Read the model definition and answer for the solid it produces. Units are mm, in the model's axes. Round coordinates to 2 decimals unless told otherwise and drop trailing zeros. Write each loop counter-clockwise with the first axis right and the second up, starting at its lowest first coordinate (ties: lowest second). Pieces come first, ordered by that corner, then holes. Notation, with made-up numbers: (53.5, 70.25) - (82.5, 70.25) arc R20 cw to (82.5, 95.25) - close; hole circle Ø10 at (45.25, -6.75). An arc over 180 degrees is marked (long way). One line per item, written item: value. Start each with the question number.
(1) Find the intervals of material crossed by L1, parallel to Y at x = -194, z = 4.25; L2, parallel to Y at x = 176.5, z = 2.75; L3, parallel to Y at x = 102.5, z = 2.75, in increasing order.
(2) Flat-ended cylindrical pins translate along their axes: pin 1 Ø1.5 at (y, z) = (-174, 6.5) entering from -X; pin 2 Ø2 at (x, z) = (-128.5, 6.5) entering from -Y; pin 3 Ø3 at (x, z) = (-5.5, 3) entering from -Y. Find the tip coordinate at first contact, or state that the pin passes through.
(3) A cutting plane is placed at A-A, the plane y = 86. Determine the outline of the cut face in (x, z).
(4) A cutting plane is placed at B-B, the plane z = 4.25. State how many separate pieces and enclosed holes the cut face has, plus the area to 3 significant figures.
(5) The mould has two halves that part along X. Classify faces 1 (the face through (58.074, 138.231, 5.051)), 2 (the face through (-52.9, 129.55, 5.05)), 3 (the face through (-3, -52, 0)): +X half, -X half, draft (parallel to the pull), parting line (faces both ways), or undercut.
(6) A cutting plane is placed at C-C, the plane y = -62. Determine the outline of the cut face in (x, z), plus the area to 3 significant figures.
from build123d import *

# Parameters (mm, degrees)
SKETCH1_R           = 250
SKETCH1_R_2         = 40
BOSS_EXTRUDE1_DEPTH = 1.6
SKETCH3_R           = 250
SKETCH3_R_2         = 240
SKETCH3_R_3         = 50
SKETCH3_R_4         = 40
BOSS_EXTRUDE2_DEPTH = 7
RIB2_REACH          = 355.658
SKETCH4_WALLS_W     = 899.315940722
SKETCH4_WALLS_H     = 10
CIRPATTERN1_COUNT   = 8
EXTRUDE_THIN1_START = -7
SKETCH5_R           = 149.934912721
SKETCH5_R_2         = 139.934912721
EXTRUDE_THIN1_DEPTH = 7


with BuildPart() as part:
    # Sketch1 → Boss-Extrude1 (new body)
    with BuildSketch(Plane.XY):
        Circle(SKETCH1_R)
        Circle(SKETCH1_R_2, mode=Mode.SUBTRACT)
    extrude(amount=BOSS_EXTRUDE1_DEPTH)

    # Sketch3 → Boss-Extrude2 (add)
    # profile 1 of 2: a face of its own
    with BuildSketch(Plane.XY.offset(1.6)):
        Circle(SKETCH3_R)
        Circle(SKETCH3_R_2, mode=Mode.SUBTRACT)
    # profile 2 of 2: a face of its own
    with BuildSketch(Plane.XY.offset(1.6)):
        Circle(SKETCH3_R_3)
        Circle(SKETCH3_R_4, mode=Mode.SUBTRACT)
    extrude(amount=BOSS_EXTRUDE2_DEPTH)

    # Sketch4 walls → Rib2 (add, up to next)
    with BuildSketch(Plane.XY.offset(8.6), mode=Mode.PRIVATE) as rib2_sk1:
        with Locations((145, 0)):
            Rectangle(SKETCH4_WALLS_W, SKETCH4_WALLS_H)
    rib2_tool1 = extrude(rib2_sk1.sketch, amount=-RIB2_REACH, mode=Mode.PRIVATE) - part.part
    rib2 = rib2_tool1.solids().sort_by_distance((145, 0, 8.6))[0]
    add(rib2)

    # CirPattern1: Rib2 ×8 about axis
    cirpattern1_axis = Axis((0, 0, 0), (0, 0, 1))
    for i in range(1, CIRPATTERN1_COUNT):
        add(rib2.rotate(cirpattern1_axis, i * 360 / CIRPATTERN1_COUNT))

    # Sketch5 → Extrude-Thin1 (add)
    with BuildSketch(Plane.XY.offset(8.6).offset(EXTRUDE_THIN1_START)):
        Circle(SKETCH5_R)
        Circle(SKETCH5_R_2, mode=Mode.SUBTRACT)
    extrude(amount=EXTRUDE_THIN1_DEPTH)


solid = part.part
Here are the results:
1. L1: -157.68 to -141.29, -5 to 5, 141.29 to 157.68
1. L2: -177.05 to -162.63, -5 to 5, 162.63 to 177.05
1. L3: -228.02 to -217.01, -109.57 to -95.27, -5 to 5, 95.27 to 109.57, 217.01 to 228.02
2. pin 1: x = -180.23
2. pin 2: y = -215.04
2. pin 3: y = -249.97
3. outline: (-234.74, 0) - (234.74, 0) - (234.74, 8.6) - (224.06, 8.6) - (224.06, 1.6) - (122.82, 1.6) - (122.82, 8.6) - (110.39, 8.6) - (110.39, 1.6) - (93.07, 1.6) - (93.07, 8.6) - (78.93, 8.6) - (78.93, 1.6) - (5, 1.6) - (5, 8.6) - (-5, 8.6) - (-5, 1.6) - (-78.93, 1.6) - (-78.93, 8.6) - (-93.07, 8.6) - (-93.07, 1.6) - (-110.39, 1.6) - (-110.39, 8.6) - (-122.82, 8.6) - (-122.82, 1.6) - (-224.06, 1.6) - (-224.06, 8.6) - (-234.74, 8.6) - close
4. separate pieces: 1
4. enclosed holes: 17
4. area: 41,700 mm²
5. face 1: undercut
5. face 2: undercut
5. face 3: draft
6. outline: (-242.19, 0) - (242.19, 0) - (242.19, 8.6) - (231.85, 8.6) - (231.85, 1.6) - (136.52, 1.6) - (136.52, 8.6) - (125.45, 8.6) - (125.45, 1.6) - (69.07, 1.6) - (69.07, 8.6) - (54.93, 8.6) - (54.93, 1.6) - (5, 1.6) - (5, 8.6) - (-5, 8.6) - (-5, 1.6) - (-54.93, 1.6) - (-54.93, 8.6) - (-69.07, 8.6) - (-69.07, 1.6) - (-125.45, 1.6) - (-125.45, 8.6) - (-136.52, 8.6) - (-136.52, 1.6) - (-231.85, 1.6) - (-231.85, 8.6) - (-242.19, 8.6) - close
6. area: 1,340 mm²
